Drawing for the job (mm, zero at the part's lowest x, y, z). A direction names the side the tool comes from. Give positions to 0.01 mm unless a question says otherwise; leave off trailing zeros. Loops run counter-clockwise (first coordinate to the right, second up) from the corner with the lowest first, then second, coordinate; pieces in that order, holes last. Notation, with made-up numbers: M 6.25,79 L 60.25,79 A14 ccw 60.25,89 Z; hole C 9.5,45 d7. An arc over 180 degrees is marked long. Use CSV: the item, a comma, the result in double quotes. Start each with the question number.
(1) Two-plate mould, pull along Z, no slides. Class the marked faces 1, 2 and 3: pulls with the +Z half, pulls with the -Z half, needs draft (parallel to the pull), parting line crosses it, or undercut.
(2) Tool access for the marked faces 4 and 5: list every direction of +Z, -Z, +X, -X, +Y, -Y with a clear straight run to the whole face (end or side of a thin tool).
(3) Flat gauge pin, fed straight in: P1, Ø6, axis at y = 16, z = 18.5, coming from the -X side. Where does the tip first touch, or does it go through?
(4) Slice it at A-A on y = 27.25. List the corners of the cut face in (x, z).
(5) Slice it at D-D on y = 7.25. List the corners of the cut face in (x, z), and give its area (3 significant figures).
(6) Wall check: line 1 along X through (y, z) = (3.75, 3.5). Give the ranges that are in metal, low to high. Write a range as from..to.
(7) Slice it at C-C on x = 8.25. List the corners of the cut face in (y, z).
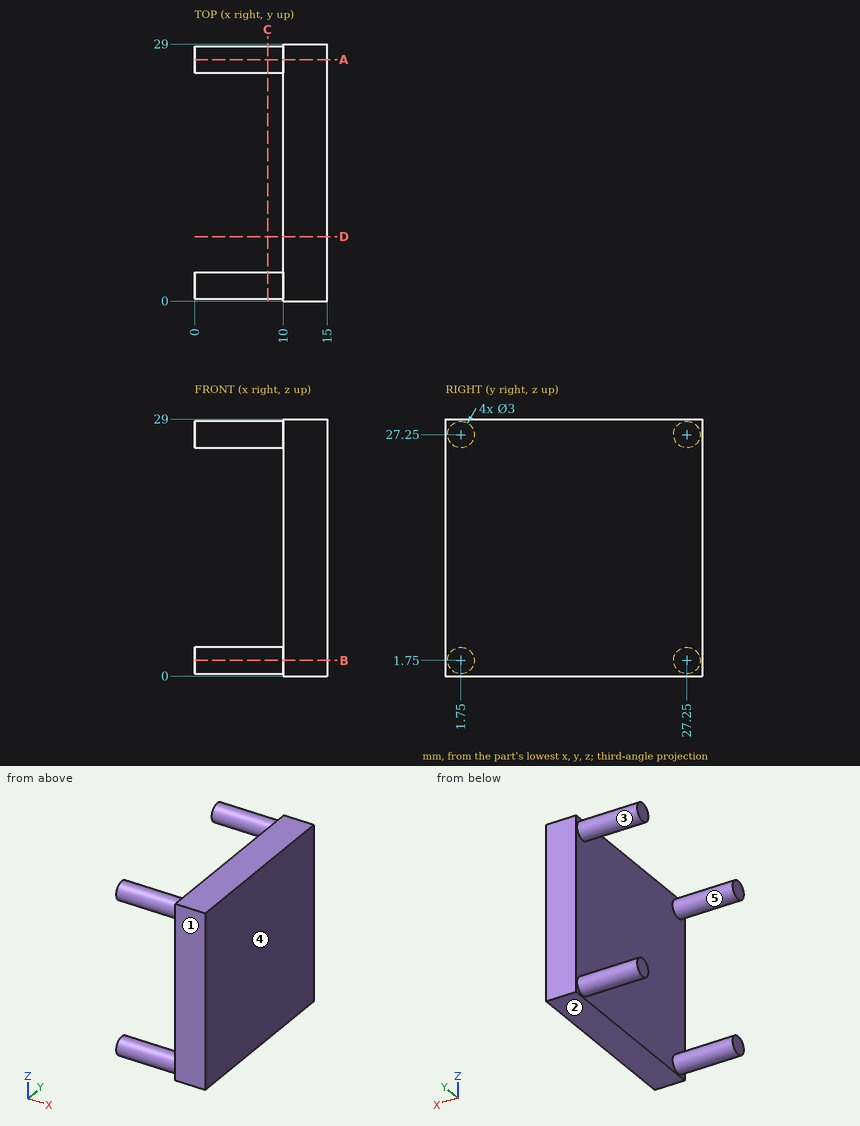
Reply:
1,face 1,"needs draft"
1,face 2,"pulls with the -Z half"
1,face 3,"undercut"
2,face 4,"+Z, -Z, +X, +Y, -Y"
2,face 5,"-X"
3,P1,"stops at x = 10"
4,outline,"M 0,0.25 L 10,0.25 L 10,0 L 15,0 L 15,29 L 10,29 L 10,28.75 L 0,28.75 L 0,25.75 L 10,25.75 L 10,3.25 L 0,3.25 Z"
5,outline,"M 10,0 L 15,0 L 15,29 L 10,29 Z"
5,area,"145 mm^2"
6,line 1,"x = 10..15"
7,outline,"C 1.75,1.75 d3; C 1.75,27.25 d3; C 27.25,1.75 d3; C 27.25,27.25 d3"
